For this review, take the finished solid that the model builds, in its own axes (mm). Face numbers are marked on the shaded views. Give positions to 0.01 mm unless a question says otherwise; leave off trailing zeros. Order: outer loops, then holes, each group sorted by start corner. A loop starts at its lowest first (then second) coordinate and runs counter-clockwise, first axis right, second up.
from build123d import *

# Parameters (mm, degrees)
SKETCH1_R           = 69
SKETCH1_R_2         = 26.5
BOSS_EXTRUDE1_DEPTH = 10
CUT_EXTRUDE1_DEPTH  = 4.5
SKETCH3_W           = 15
SKETCH3_H           = 8
CUT_EXTRUDE2_DEPTH  = 99.091793744
SKETCH4_R           = 1.25
CUT_EXTRUDE3_DEPTH  = 99.091793744
SKETCH5_R           = 2.75
CUT_EXTRUDE4_DEPTH  = 8.2


with BuildPart() as part:
    # Sketch1 → Boss-Extrude1 (new body)
    with BuildSketch(Plane(origin=(0, 0, 0), x_dir=(1, 0, 0), z_dir=(0, 1, 0))):
        with Locations(Location((0, 0, 0), (0, 0, 270))):
            Circle(SKETCH1_R)
        with Locations(Location((0, 0, 0), (0, 0, 270))):
            Circle(SKETCH1_R_2, mode=Mode.SUBTRACT)
    extrude(amount=BOSS_EXTRUDE1_DEPTH)

    # Sketch2 → Cut-Extrude1 (cut)
    with BuildSketch(Plane.XZ):
        Polygon((-13, -34.242640687), (-17.242640687, -30), (-13, -25.757359313), (-8.757359313, -30), align=None)
        Polygon((-35.46, -58.000880986), (-39.702640687, -53.758240299), (-35.46, -49.515599611), (-31.217359313, -53.758240299), align=None)
        Polygon((13, -34.242640687), (8.757359313, -30), (13, -25.757359313), (17.242640687, -30), align=None)
        Polygon((35.46, -58.000880986), (31.217359313, -53.758240299), (35.46, -49.515599611), (39.702640687, -53.758240299), align=None)
    extrude(amount=-CUT_EXTRUDE1_DEPTH, mode=Mode.SUBTRACT)

    # Sketch3 → Cut-Extrude2 (cut, through all)
    with BuildSketch(Plane.XZ):
        with Locations((0, -51.875)):
            Rectangle(SKETCH3_W, SKETCH3_H)
    extrude(amount=-CUT_EXTRUDE2_DEPTH, mode=Mode.SUBTRACT)

    # Sketch4 → Cut-Extrude3 (cut, through all)
    with BuildSketch(Plane.XZ):
        with Locations(Location((-13, -30, 0), (0, 0, 270))):
            Circle(SKETCH4_R)
        with Locations(Location((13, -30, 0), (0, 0, 270))):
            Circle(SKETCH4_R)
        with Locations(Location((-35.46, -53.758240299, 0), (0, 0, 270))):
            Circle(SKETCH4_R)
        with Locations(Location((35.46, -53.758240299, 0), (0, 0, 270))):
            Circle(SKETCH4_R)
    extrude(amount=-CUT_EXTRUDE3_DEPTH, mode=Mode.SUBTRACT)

    # Sketch5 → Cut-Extrude4 (cut)
    with BuildSketch(Plane.XZ):
        with Locations(Location((-44.901280605, 44.901280605, 0), (0, 0, 270))):
            Circle(SKETCH5_R)
        with Locations(Location((44.901280605, 44.901280605, 0), (0, 0, 270))):
            Circle(SKETCH5_R)
        with Locations(Location((-43, -46.725260834, 0), (0, 0, 270))):
            Circle(SKETCH5_R)
        with Locations(Location((43, -46.725260834, 0), (0, 0, 270))):
            Circle(SKETCH5_R)
    extrude(amount=-CUT_EXTRUDE4_DEPTH, mode=Mode.SUBTRACT)


solid = part.part
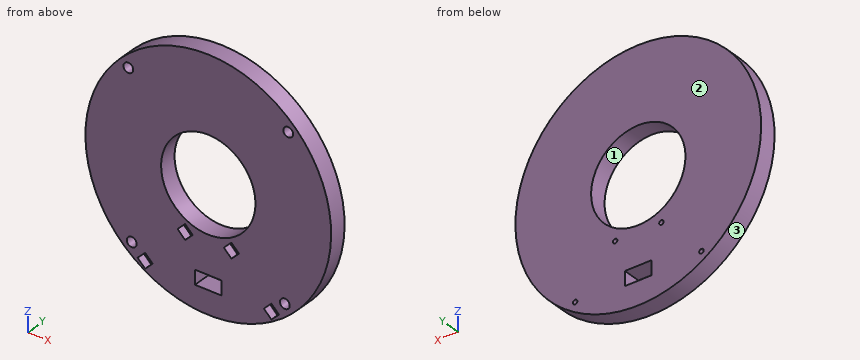
1) We need section C-C on z = -23. Give the boundary of the cut face in (x, y), then the cut area to 3 significant figures.
Answer sheet:
outline: (-65.05, 0) - (-13.16, 0) - (-13.16, 10) - (-65.05, 10) - close; (13.16, 0) - (65.05, 0) - (65.05, 10) - (13.16, 10) - close
area: 1,040 mm2
2) We need section B-B on z = 0. Give the boundary of the cut face in (x, y), then the cut area to 3 significant figures.
Answer sheet:
outline: (-69, 0) - (-26.5, 0) - (-26.5, 10) - (-69, 10) - close; (26.5, 0) - (69, 0) - (69, 10) - (26.5, 10) - close
area: 850 mm2
3) We need section D-D on z = -38.5. Give the boundary of the cut face in (x, y).
Answer sheet:
outline: (-57.26, 0) - (57.26, 0) - (57.26, 10) - (-57.26, 10) - close
4) Clearance check with flat-ended pins moving along their axes: pin 1 (5 mm diameter, centred on x = 0.5, y = 7, fed in from -Z); pin 2 (4 mm diameter, centred on y = 3.5, z = -50, fed in from +X); pin 3 (5 mm diameter, centred on y = 7.5, z = 22.5, fed in from -X); pin 4 (3 mm diameter, centred on x = -46, z = 44.5, fed in from -Y). State where each tip first meets the part, or that it passes through.
Answer sheet:
pin 1: stops at z = -69
pin 2: stops at x = 49.57
pin 3: stops at x = -66.04
pin 4: stops at y = 8.2
5) Draft analysis for pull direction X (two halves, no side actions). For the marked faces 1, 2 and 3, state which applies: +X half, -X half, draft (parallel to the pull), parting line (faces both ways), or undercut.
Answer sheet:
face 1: undercut
face 2: draft
face 3: parting line
6) We need section A-A on x = 0. Give the boundary of the cut face in (y, z) (3 decimals).
Answer sheet:
outline: (0, -69) - (10, -69) - (10, -55.875) - (0, -55.875) - close; (0, -47.875) - (10, -47.875) - (10, -26.5) - (0, -26.5) - close; (0, 26.5) - (10, 26.5) - (10, 69) - (0, 69) - close
7) To check wall thickness, follow line 1 (X direction, y = 3.25, z = -57); line 2 (X direction, y = 2, z = -31); line 3 (Z direction, x = -45, y = 7.75). State the ranges of each line that lie inside material, in increasing order.
Answer sheet:
line 1: x = -38.88 to -36.46, -34.46 to 34.46, 36.46 to 38.88
line 2: x = -61.64 to -16.24, -9.76 to 9.76, 16.24 to 61.64
line 3: z = -52.31 to -48.61, -44.84 to 42.15, 47.65 to 52.31
